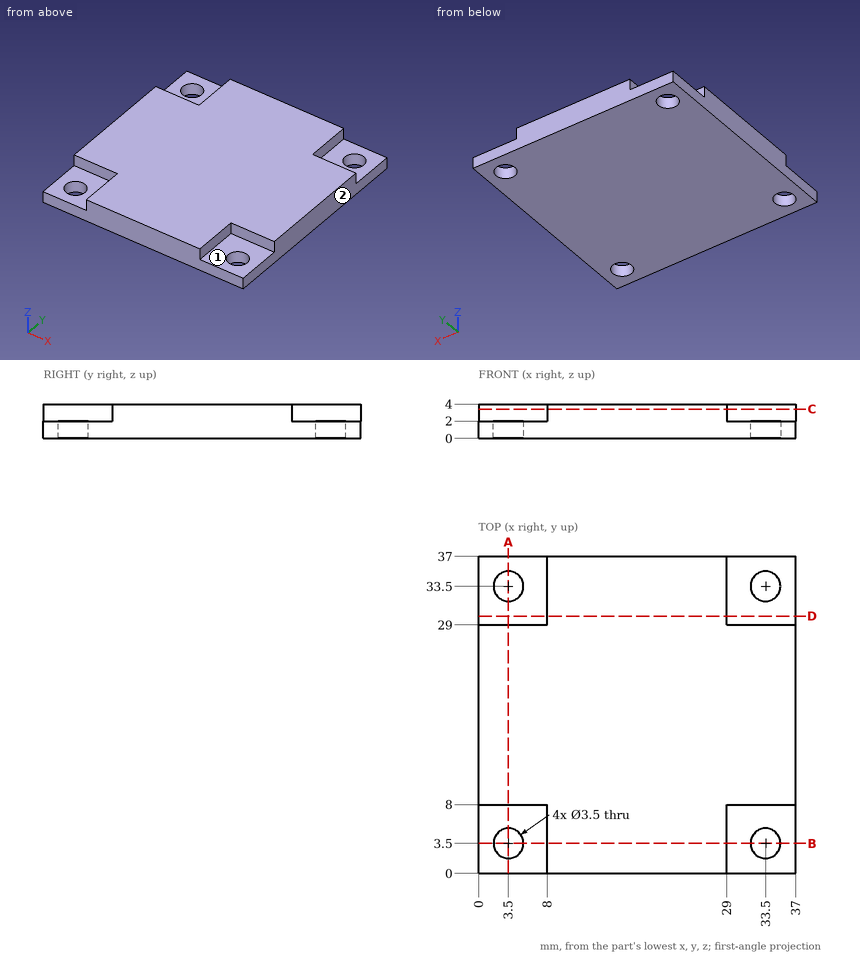
Input: dimensioned drawing with shaded views. Units: mm. Origin: part minimum x, y, z. A direction names the side the tool comes from. Coordinates: 2 decimals unless noted, no trailing zeros. Write each loop counter-clockwise with the first axis right and the second up, starting at its lowest first coordinate (ties: lowest second). Pieces come first, ordered by that corner, then holes. Notation, with made-up numbers: M 38.25,77 L 62.25,77 A19 cw 62.25,100 Z; hole C -26,-24 d4. An arc over 180 degrees is marked long. Use one line per item in the form item = value.
Q1. Section C-C (z = 3.4). Return loops of the section in (x, y).
Answer below:
outline = M 0,8 L 8,8 L 8,0 L 29,0 L 29,8 L 37,8 L 37,29 L 29,29 L 29,37 L 8,37 L 8,29 L 0,29 Z
Q2. First-contact query: pin 1 (4 mm diameter, centred on x = 32, y = 5.5, fed in from +Z); pin 2 (1.6 mm diameter, centred on x = 32.5, z = 3, fed in from -Y); pin 3 (1 mm diameter, centred on y = 3.5, z = 3, fed in from +X); pin 4 (2 mm diameter, centred on x = 33.5, y = 33.5, fed in from +Z). Flat tips, straight axial feed; report the tip coordinate or a pass-through.
Answer below:
pin_1 = 2
pin_2 = 8
pin_3 = 29
pin_4 = through
Q3. Section D-D (y = 30). Return loops of the section in (x, z).
Answer below:
outline = M 0,0 L 37,0 L 37,2 L 29,2 L 29,4 L 8,4 L 8,2 L 0,2 Z
Q4. Section A-A (x = 3.5). Return loops of the section in (y, z).
Answer below:
outline = M 0,0 L 1.75,0 L 1.75,2 L 0,2 Z; M 5.25,0 L 31.75,0 L 31.75,2 L 29,2 L 29,4 L 8,4 L 8,2 L 5.25,2 Z; M 35.25,0 L 37,0 L 37,2 L 35.25,2 Z
Q5. Material intervals for probe 1 along Y at (x, z) = (3.5, 1.6); probe 2 along Y at (x, z) = (35, 1); probe 3 along X at (y, z) = (32.5, 0.9), sorted ascending. Write a range as from..to.
Answer below:
probe_1 = 0..1.75, 5.25..31.75, 35.25..37
probe_2 = 0..2.6, 4.4..32.6, 34.4..37
probe_3 = 0..2.06, 4.94..32.06, 34.94..37
Q6. Set-up query: the marked faces 1 and 2. Return all of +Z, -Z, +X, -X, +Y, -Y with unobstructed straight access to the full face (end or side cutting, diameter ignored); none if empty.
Answer below:
face_1 = +Z, +X, -Y
face_2 = +Z, -Z, +X, +Y, -Y
